Could you check a few things on this model? Use its own coordinates, in mm. A direction names the side the tool comes from. Give positions to 0.01 mm unless a question says otherwise; leave off trailing zeros. Order: outer loops, then holes, each group sorted by start corner. A loop starts at its lowest first (then second) coordinate and runs counter-clockwise, first axis right, second up.
from build123d import *

# Parameters (mm, degrees)
F0_W          = 30
F0_H          = 33
F1_DEPTH      = 22
F2_W          = 20
F2_H          = 4.4
F3_DEPTH      = 30.001
F4_R          = 2
F5_DEPTH      = 5
F5_DEPTH_BACK = 20.001
F6_DEPTH      = 13.001
F7_R          = 2
F8_DEPTH      = 10.601
F9_DEPTH      = 3.5
F10_R         = 1


with BuildPart() as f1:
    # F0 (on Top) → F1 (new body)
    with BuildSketch(Plane.XY):
        Rectangle(F0_W, F0_H)
    extrude(amount=F1_DEPTH)

    # F2 (on face) → F3 (cut, through all)
    with BuildSketch(Plane.YZ.offset(15)):
        with Locations((-6.5, 9.2)):
            Rectangle(F2_W, F2_H)
    extrude(amount=-F3_DEPTH, mode=Mode.SUBTRACT)

    # F4 (on face) → F5 (cut, two sides)
    with BuildSketch(Plane.XZ.offset(-3.5)) as f5_sk:
        Polygon((-2.7135462652, 11.4), (2.7135462652, 11.4), (2.0207259422, 12.6), (-2.0207259422, 12.6), align=None)
        Polygon((-2.829016319, 7), (2.829016319, 7), (4.0414518843, 9.1), (2.7135462652, 11.4), (-2.7135462652, 11.4), (-4.0414518843, 9.1), align=None)
        with Locations((0, 9.1)):
            Circle(F4_R, mode=Mode.SUBTRACT)
        Polygon((-2.0207259422, 5.6), (2.0207259422, 5.6), (2.829016319, 7), (-2.829016319, 7), align=None)
    extrude(amount=-F5_DEPTH, mode=Mode.SUBTRACT)
    extrude(f5_sk.sketch, amount=F5_DEPTH_BACK, mode=Mode.SUBTRACT)

    # F6 (cut, through all): a face of the model
    f6_faces = [f1.faces().sort_by_distance(p)[0] for p in [
        (0, 3.5, 9.1),
    ]]
    extrude(f6_faces, amount=-F6_DEPTH, mode=Mode.SUBTRACT)

    # F7 (on face) → F8 (cut, through all)
    with BuildSketch(Plane(origin=(0, 0, 11.4), x_dir=(1, 0, 0), z_dir=(0, 0, -1))):
        with Locations((0, 6.5)):
            Circle(F7_R)
    extrude(amount=-F8_DEPTH, mode=Mode.SUBTRACT)

    # F7 (on face) → F9 (cut)
    with BuildSketch(Plane(origin=(0, 0, 11.4), x_dir=(1, 0, 0), z_dir=(0, 0, -1))):
        Polygon((-4.0414518843, 6.5), (-2.7135462652, 4.2), (-2.7135462652, 8.8), align=None)
        Polygon((-2.7135462652, 8.8), (-2.7135462652, 4.2), (-2.0207259422, 3), (2.0207259422, 3), (2.7135462652, 4.2), (2.7135462652, 8.8), (2.0207259422, 10), (-2.0207259422, 10), align=None)
        with Locations((0, 6.5)):
            Circle(F7_R, mode=Mode.SUBTRACT)
        Polygon((2.7135462652, 8.8), (2.7135462652, 4.2), (4.0414518843, 6.5), align=None)
    extrude(amount=-F9_DEPTH, mode=Mode.SUBTRACT)

    # F10
    f10_edges = [f1.edges().sort_by_distance(p)[0] for p in [
        (0, 16.5, 0),
        (15, 16.5, 11),
        (0, 16.5, 22),
        (-15, 16.5, 11),
        (-15, 0, 0),
        (0, -16.5, 0),
        (15, 0, 0),
        (-15, 0, 22),
        (0, -16.5, 22),
        (15, 0, 22),
        (-15, -16.5, 3.5),
        (-15, -16.5, 16.7),
        (15, -16.5, 3.5),
        (15, -16.5, 16.7),
        (15, -6.5, 11.4),
        (15, -6.5, 7),
        (8.914508, -16.5, 7),
        (-8.914508, -16.5, 7),
        (-8.856773, -16.5, 11.4),
        (-15, 3.5, 9.2),
        (-15, -6.5, 7),
        (-15, -6.5, 11.4),
        (15, 3.5, 9.2),
    ]]
    fillet(f10_edges, radius=F10_R)


solid = f1.part
Item 1: Imagine slicing it at A-A on y = -1. List the corners of the cut face in (x, z) for me.
Findings:
outline: (-15, 1) arc R1 ccw to (-14, 0) - (14, 0) arc R1 ccw to (15, 1) - (15, 6) arc R1 ccw to (14, 7) - (2.83, 7) - (2.02, 5.6) - (-2.02, 5.6) - (-2.83, 7) - (-14, 7) arc R1 ccw to (-15, 6) - close; (-15, 12.4) arc R1 ccw to (-14, 11.4) - (-2.71, 11.4) - (-2.02, 12.6) - (2.02, 12.6) - (2.71, 11.4) - (14, 11.4) arc R1 ccw to (15, 12.4) - (15, 21) arc R1 ccw to (14, 22) - (-14, 22) arc R1 ccw to (-15, 21) - close
Item 2: For faces 5 (the flat face through (8, 3.5, 9)), 6 (the cylindrical face through (-14.715, 3.801, 9.155)), 7 (the cylindrical face through (-0.26, -8.483, 18.4)), which set-ups out of +Z, -Z, +X, -X, +Y, -Y let a thin tool reach every point of the face, with its end or its side?
Findings:
face 5: +X, -X, -Y
face 6: -X, -Y
face 7: +Z
Item 3: We'd pull the mould along X, two halves only. Please class faces 1 (the cylindrical face through (14.715, -5.853, 11.701)), 2 (the flat face through (0, -13, 12.6)), 3 (the flat face through (0, -16.5, 16)), 4 (the cylindrical face through (-14.715, -5.64, 6.699)): +X half, -X half, draft (parallel to the pull), parting line (faces both ways), or undercut.
Findings:
face 1: +X half
face 2: undercut
face 3: draft
face 4: -X half
Item 4: For pin 1 (1.3 mm diameter, centred on x = 9, z = 8.5, fed in from -Y); pin 2 (3.5 mm diameter, centred on x = 0, y = -6.5, fed in from +Z); pin 3 (5 mm diameter, centred on x = 0, z = 9.1, fed in from -Y), each with a flat end and sliding along its axis, tell me the tip position at first contact or that it passes through.
Findings:
pin 1: stops at y = 3.5
pin 2: stops at z = 5.6
pin 3: stops at y = 8.5
Item 5: Imagine slicing it at B-B on x = -10.5. List the corners of the cut face in (y, z) for me, then the cut area to 3 significant figures.
Findings:
outline: (-16.5, 1) arc R1 ccw to (-15.5, 0) - (15.5, 0) arc R1 ccw to (16.5, 1) - (16.5, 21) arc R1 ccw to (15.5, 22) - (-15.5, 22) arc R1 ccw to (-16.5, 21) - (-16.5, 12.4) arc R1 ccw to (-15.5, 11.4) - (3.5, 11.4) - (3.5, 7) - (-15.5, 7) arc R1 ccw to (-16.5, 6) - close
area: 637 mm2
Item 6: Imagine slicing it at C-C on z = 10. List the corners of the cut face in (x, y) for me, then the cut area to 3 significant figures.
Findings:
outline: (-15, 4.5) arc R1 ccw to (-14, 3.5) - (-3.52, 3.5) - (-3.52, 8.5) - (-1.79, 8.5) - (-1.79, 16.5) - (-14, 16.5) arc R1 ccw to (-15, 15.5) - close; (1.79, 8.5) - (3.52, 8.5) - (3.52, 3.5) - (14, 3.5) arc R1 ccw to (15, 4.5) - (15, 15.5) arc R1 ccw to (14, 16.5) - (1.79, 16.5) - close
area: 325 mm2
Item 7: Imagine slicing it at D-D on x = 0. List the corners of the cut face in (y, z) for me, then the cut area to 3 significant figures.
Findings:
outline: (-16.5, 1) arc R1 ccw to (-15.5, 0) - (15.5, 0) arc R1 ccw to (16.5, 1) - (16.5, 7.1) - (8.5, 7.1) - (8.5, 5.6) - (-16.5, 5.6) - close; (-16.5, 12.6) - (-10, 12.6) - (-10, 14.9) - (-8.5, 14.9) - (-8.5, 22) - (-15.5, 22) arc R1 ccw to (-16.5, 21) - close; (-4.5, 14.9) - (-3, 14.9) - (-3, 12.6) - (8.5, 12.6) - (8.5, 11.1) - (16.5, 11.1) - (16.5, 21) arc R1 ccw to (15.5, 22) - (-4.5, 22) - close
area: 474 mm2
Item 8: Please list where these lines run through material, in increasing order: line 1 along Y through (x, z) = (0, 18.5); line 2 along Z through (x, y) = (1.5, -8); line 3 along Z through (x, y) = (-5, -8).
Findings:
line 1: y = -16.5 to -8.5, -4.5 to 16.5
line 2: z = 0 to 5.6, 14.9 to 22
line 3: z = 0 to 7, 11.4 to 22
